For this review, use the dimensioned drawing (mm, ordinates from the lowest corner) and the shaded views. Round coordinates to 2 decimals unless told otherwise and drop trailing zeros. Loops run counter-clockwise (first coordinate to the right, second up) from the corner with the lowest first, then second, coordinate; pieces in that order, holes last. Notation, with made-up numbers: (15, 62.5) - (49, 62.5) arc R11 ccw to (49, 79.5) - close; hole circle Ø1 at (36, 75.5). An arc over 180 degrees is marked (long way). Use one line per item in the form item = value. Start each with the question number.
(1) We need section B-B, the plane x = 21.5. Write out the cut boundary in (y, z).
(2) We need section D-D, the plane z = 28. Write out the cut boundary in (x, y), then the cut area to 3 significant figures.
(3) Wall thickness on probe 1 along Z at (x, y) = (38, 1.55); probe 2 along X at (y, z) = (2.75, 9.5); probe 3 along Z at (x, y) = (15, 0.95): over which ranges is each line inside the solid? List them lowest first. Write a range as [from, to].
(4) For pin 1 (12 mm diameter, centred on x = 23.5, z = 30, fed in from +Y); pin 2 (1.7 mm diameter, centred on y = 1, z = 22.5, fed in from +X); pin 3 (1.5 mm diameter, centred on y = 0.5, z = 9, fed in from +X); pin 4 (1 mm diameter, centred on y = 1.5, z = 29.5, fed in from +X), all flat-tipped, find the tip position at first contact; note any pin that passes through.
(5) We need section A-A, the plane x = 38. Write out the cut boundary in (y, z), then the cut area to 3 significant figures.
(6) We need section C-C, the plane z = 39.5. Write out the cut boundary in (x, y), then the cut area to 3 significant figures.
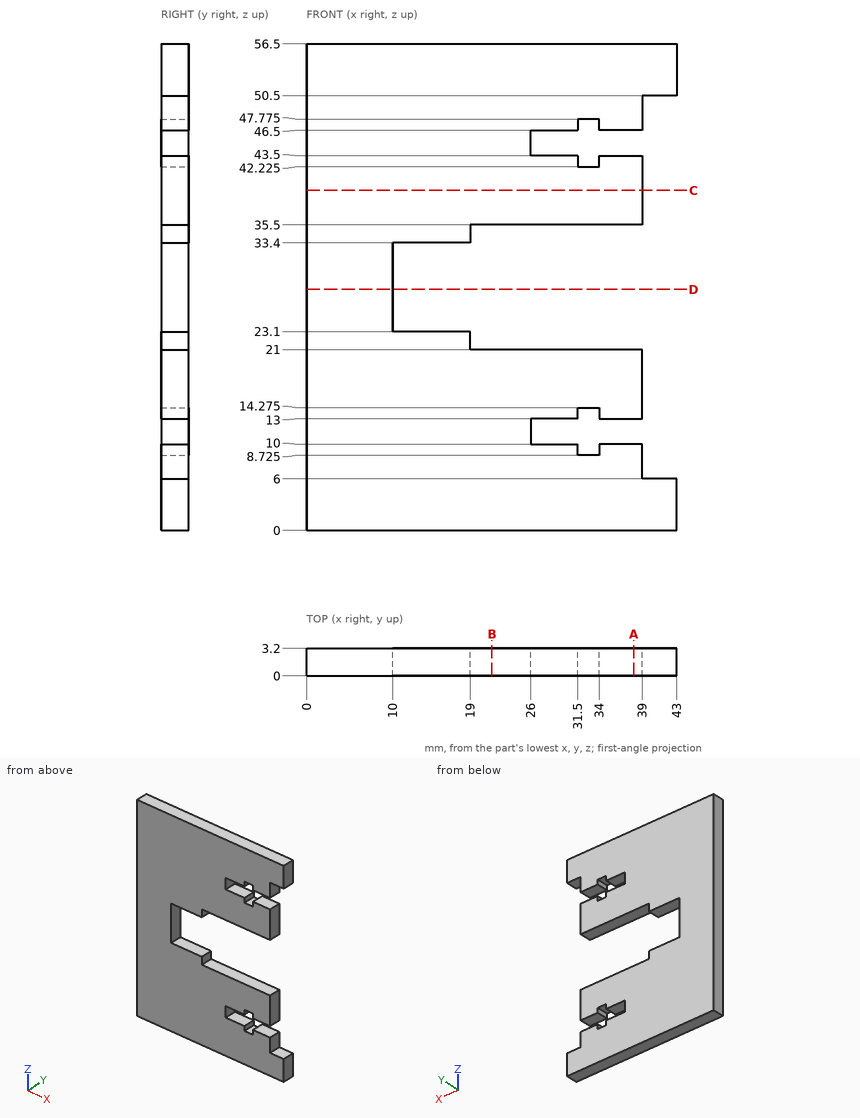
Data:
q1.outline = (0, 0) - (3.2, 0) - (3.2, 21) - (0, 21) - close; (0, 35.5) - (3.2, 35.5) - (3.2, 56.5) - (0, 56.5) - close
q2.outline = (0, 0) - (10, 0) - (10, 3.2) - (0, 3.2) - close
q2.area = 32.0 mm^2
q3.probe_1 = [0, 10], [13, 21], [35.5, 43.5], [46.5, 56.5]
q3.probe_2 = [0, 31.5], [34, 39]
q3.probe_3 = [0, 23.1], [33.4, 56.5]
q4.pin_1 = 3.2
q4.pin_2 = 19
q4.pin_3 = 39
q4.pin_4 = 10
q5.outline = (0, 0) - (3.2, 0) - (3.2, 10) - (0, 10) - close; (0, 13) - (3.2, 13) - (3.2, 21) - (0, 21) - close; (0, 35.5) - (3.2, 35.5) - (3.2, 43.5) - (0, 43.5) - close; (0, 46.5) - (3.2, 46.5) - (3.2, 56.5) - (0, 56.5) - close
q5.area = 115 mm^2
q6.outline = (0, 0) - (39, 0) - (39, 3.2) - (0, 3.2) - close
q6.area = 125 mm^2
